from build123d import *

# Parameters (mm, degrees)
F0_R        = 12.5
F1_DEPTH    = 9
F2_R        = 6.25
F3_DEPTH    = 4
F4_R        = 2
F5_DEPTH    = 1.5
F6_R        = 1
F7_S5_R     = 2
F7_T6_DEPTH = 21


# Not quite as in the source:
# - a fillet or chamfer that OpenCascade refuses, or shapes differently, is made with other operations: its cross-section is extruded or revolved along the edge and cut away or added


with BuildPart() as f1:
    # F0 (on Top) → F1 (new body)
    with BuildSketch(Plane.XY):
        Circle(F0_R)
        with BuildLine():
            ThreePointArc((-3.35, 0), (-1.7058759905, 2.8831384124), (1.6126788687, 2.9362845343))
            Line((1.6126788687, 2.9362845343), (1.6126788687, 0))
            Line((1.6126788687, 0), (1.6126788687, -2.9362845343))
            ThreePointArc((1.6126788687, -2.9362845343), (-1.7058759905, -2.8831384124), (-3.35, 0))
        make_face(mode=Mode.SUBTRACT)
    extrude(amount=F1_DEPTH)

    # F2 (on face) → F3 (cut)
    with BuildSketch(Plane(origin=(0, 0, 0), x_dir=(1, 0, 0), z_dir=(0, 0, -1))):
        with Locations((0, -0.4813171179)):
            Circle(F2_R)
    extrude(amount=-F3_DEPTH, mode=Mode.SUBTRACT)

    # F4 (on face) → F5 (join)
    with BuildSketch(Plane.XY.offset(9)):
        with Locations((-10, 0)):
            Circle(F4_R)
    extrude(amount=F5_DEPTH)

    # F6
    f6_edges = [f1.edges().sort_by_distance(p)[0] for p in [
        (-12, 0, 10.5),
    ]]
    fillet(f6_edges, radius=F6_R)

    # F7: fillet of radius 3 on 1 edges, made by hand


with BuildPart() as f7_tool2:
    # F7_s3 → F7_t4 (revolve)
    with BuildSketch(Plane.XZ):
        with BuildLine():
            ThreePointArc((9.5, 9), (11.6213203436, 8.1213203436), (12.5, 6))
            Line((12.5, 6), (12.5, 9))
            Line((12.5, 9), (9.5, 9))
        make_face()
    revolve(axis=Axis((0, 0, 9), (0, 0, 1)))

    # F7_s5 → F7_t6 (cut, symmetric)
    with BuildSketch(Plane.XY.offset(6.4)):
        with Locations((-10, 0)):
            Circle(F7_S5_R)
    extrude(amount=F7_T6_DEPTH, both=True, mode=Mode.SUBTRACT)


with BuildPart() as f1_1:
    add(f1.part)

    # F7_t1: cut F7_tool2
    add(f7_tool2.part, mode=Mode.SUBTRACT)


solid = f1_1.part
Work out the finished part from the listing and answer in its coordinate system (mm). A direction names the side the tool comes from. Coordinates: 2 decimals unless noted, no trailing zeros. Write each loop counter-clockwise with the first axis right and the second up, starting at its lowest first coordinate (ties: lowest second). Pieces come first, ordered by that corner, then holes.
1. For a pull along X with two mould halves and no side action, classify faces 5 (the flat face through (2, 0, 9)), 6 (the flat face through (3, 0, 4)), 7 (the cylindrical face through (11.923, 3.755, 2.958)) as +X half, -X half, draft (parallel to the pull), parting line (faces both ways), or undercut.
Results list:
face 5: draft
face 6: undercut
face 7: parting line
2. The part is cut by section B-B, the plane z = 1.25. Write down the section's boundary in (x, y), and give its area (3 significant figures).
Results list:
outline: circle Ø25 at (0, 0); hole circle Ø12.5 at (0, 0.48)
area: 368 mm2
3. Flat-ended cylindrical pins translate along their axes: pin 1 (1 mm diameter, centred on x = 1.5, y = -6, fed in from -Z); pin 2 (6 mm diameter, centred on x = 1.5, y = 2, fed in from -Z); pin 3 (10 mm diameter, centred on x = 5, y = -5.5, fed in from +Z); pin 4 (2 mm diameter, centred on y = 8.5, z = 5.5, fed in from -X). Find the tip coordinate at first contact, or state that the pin passes through.
Results list:
pin 1: stops at z = 0
pin 2: stops at z = 4
pin 3: stops at z = 9
pin 4: stops at x = -10
4. The part is cut by section A-A, the plane x = 0. Write down the section's boundary in (y, z), and give its area (3 significant figures).
Results list:
outline: (-12.5, 0) - (-5.77, 0) - (-5.77, 4) - (-3.35, 4) - (-3.35, 9) - (-9.5, 9) arc R3 ccw to (-12.5, 6) - close; (3.35, 4) - (6.73, 4) - (6.73, 0) - (12.5, 0) - (12.5, 6) arc R3 ccw to (9.5, 9) - (3.35, 9) - close
area: 138 mm2
5. Consider line 1 along Y through (x, z) = (0, 1.75); line 2 along Y through (x, z) = (0.5, 7); line 3 along Z through (x, y) = (4, -1). Determine where each line is inside the solid, lowest interval first.
Results list:
line 1: y = -12.5 to -5.77, 6.73 to 12.5
line 2: y = -12.32 to -3.31, 3.31 to 12.32
line 3: z = 4 to 9
6. For faces 1 (the cylindrical face through (-12, 0, 9)), 2 (the cylindrical face through (5.96, -1.4, 1.97)), 3 (the flat face through (2.6, -5.4, 0)), 4 (the flat face through (1.613, 0, 6)), determine the directions among +Z, -Z, +X, -X, +Y, -Y from which every point of the face is accessible in a straight line to the end or side of a thin tool.
Results list:
face 1: +Z
face 2: -Z
face 3: -Z, +X, -X, +Y, -Y
face 4: +Z, -Z
